Input: part model. Units: mm. Frame: model coordinates. Face numbers are marked on the shaded views. A direction names the side the tool comes from. Give positions to 0.01 mm unless a question says otherwise; leave off trailing zeros. Loops run counter-clockwise (first coordinate to the right, second up) from the corner with the lowest first, then second, coordinate; pieces in that order, holes last. Notation, with made-up numbers: M 42,39 L 65,39 A21 ccw 65,70 Z; hole C 30.5,-0.75 d8. An arc over 180 degrees is marked long. Answer as a JSON object with one key per item and string values. Group by question number.
```python
from build123d import *

# Parameters (mm, degrees)
F0_R     = 12.5
F1_DEPTH = 50
F3_DEPTH = 12.5
F5_DEPTH = 10
F7_DEPTH = 2


with BuildPart() as f1:
    # F0 (on Right) → F1 (new body, symmetric)
    with BuildSketch(Plane.YZ):
        Circle(F0_R)
    extrude(amount=F1_DEPTH, both=True)

    # F2 (on Front) → F3 (join)
    with BuildSketch(Plane.XZ):
        with BuildLine():
            Line((35, 12.5), (26.5, 12.5))
            ThreePointArc((26.5, 12.5), (14, 0), (26.5, -12.5))
            Line((26.5, -12.5), (35, -12.5))
            ThreePointArc((35, -12.5), (47.5, 0), (35, 12.5))
        make_face()
    extrude(amount=F3_DEPTH)

    # F4 (on face) → F5 (join)
    with BuildSketch(Plane.XZ.offset(12.5)):
        with BuildLine():
            Line((35, 8.5), (26.5, 8.5))
            ThreePointArc((26.5, 8.5), (18, 0), (26.5, -8.5))
            Line((26.5, -8.5), (35, -8.5))
            ThreePointArc((35, -8.5), (43.5, 0), (35, 8.5))
        make_face()
    extrude(amount=F5_DEPTH)

    # F6 (on face) → F7 (join)
    with BuildSketch(Plane.XZ.offset(22.5)):
        with BuildLine():
            Line((35, 10), (26.5, 10))
            ThreePointArc((26.5, 10), (16.5, 0), (26.5, -10))
            Line((26.5, -10), (35, -10))
            ThreePointArc((35, -10), (45, 0), (35, 10))
        make_face()
    extrude(amount=F7_DEPTH)


solid = f1.part
```
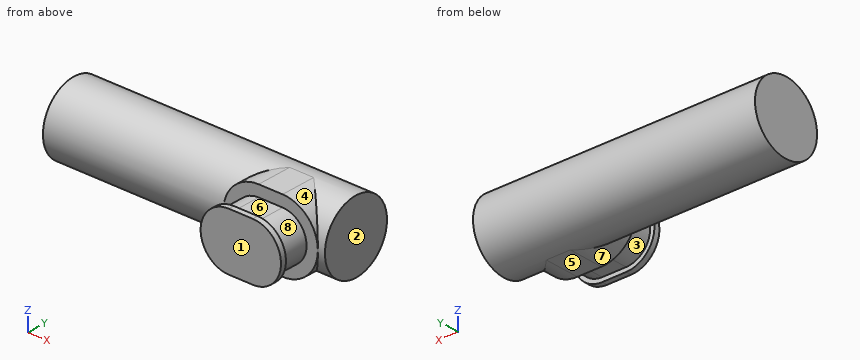
1. Material intervals for L1, parallel to Y at x = 43.5, z = -2.5; L2, parallel to Y at x = 31.5, z = 9.25; L3, parallel to X at y = -17.5, z = -4.25, sorted ascending.
2. Section A-A (x = 25). Output: boundary loops of the cut face in (y, z).
3. Section B-B (z = 6.25). Output: boundary loops of the cut face in (x, y).
4. Mould query, pull axis Y, two halves, no side actions, for the marked faces 1, 2 and 3. Classes: pulls with the +Y half, pulls with the -Y half, needs draft (parallel to the pull), parting line crosses it, or undercut.
5. First-contact query: P1, Ø3, axis at x = 3.5, z = 8.5, coming from the -Y side; P2, Ø1.5, axis at x = -19, y = 7, coming from the -Z side; P3, Ø8, axis at x = 23.5, y = 6, coming from the +Z side. Flat tips, straight axial feed; report the tip coordinate or a pass-through.
6. Reachability of the marked faces 4, 5, 6, 7 and 8 from +Z, -Z, +X, -X, +Y, -Y: full face, straight path, thin tool, end or side. Return the list, or none.
7. Section C-C (y = -3). Output: boundary loops of the cut face in (x, z).
8. Section D-D (y = 10). Output: boundary loops of the cut face in (x, z).
Geometry results:
{
 "1": {"L1": "-24.5 to -22.5, -12.5 to 12.25", "L2": "-24.5 to -22.5, -12.5 to 8.41", "L3": "19.14 to 42.36"},
 "2": {"outline": "M -24.5,-9.89 L -22.5,-9.89 L -22.5,-8.37 L -12.5,-8.37 L -12.5,-12.41 L -1.5,-12.41 A12.5 ccw long -1.5,12.41 L -12.5,12.41 L -12.5,8.37 L -22.5,8.37 L -22.5,9.89 L -24.5,9.89 Z"},
 "3": {"outline": "M -50,-10.83 L 15.67,-10.83 L 15.67,-12.5 L 20.74,-12.5 L 20.74,-22.5 L 18.69,-22.5 L 18.69,-24.5 L 42.81,-24.5 L 42.81,-22.5 L 40.76,-22.5 L 40.76,-12.5 L 45.83,-12.5 L 45.83,-10.83 L 50,-10.83 L 50,10.83 L -50,10.83 Z"},
 "4": {"face 1": "pulls with the -Y half", "face 2": "needs draft", "face 3": "undercut"},
 "5": {"P1": "y = -10.36", "P2": "z = -10.83", "P3": "z = 12.34"},
 "6": {"face 4": "+Z, +X, -Y", "face 5": "-Z, +X, -X, +Y, -Y", "face 6": "+Z, +X, -X", "face 7": "-Z, -X, -Y", "face 8": "+X"},
 "7": {"outline": "M -50,-12.13 L 23.5,-12.13 A12.5 ccw 26.5,-12.5 L 35,-12.5 A12.5 ccw 38,-12.13 L 50,-12.13 L 50,12.13 L 38,12.13 A12.5 ccw 35,12.5 L 26.5,12.5 A12.5 ccw 23.5,12.13 L -50,12.13 Z"},
 "8": {"outline": "M -50,-7.5 L 50,-7.5 L 50,7.5 L -50,7.5 Z"}
}
